Could you check a few things on this model? Use its own coordinates, in mm. Coordinates: 2 decimals unless noted, no trailing zeros. Write each loop counter-clockwise with the first axis right and the second up, starting at its lowest first coordinate (ties: lowest second). Pieces come first, ordered by that corner, then holes. Notation, with made-up numbers: M 15.25,7 L 39.25,7 A29 ccw 39.25,46 Z; hole C -31,84 d9. An arc over 180 degrees is marked long. Answer as CSV lines item,"result". Start each with the question number.
Item 1: We'd pull the mould along X, two halves only. Please class faces 1 (the cylindrical face through (137.02, -138.517, -0.744)), 2 (the cylindrical face through (137.528, -164.615, -0.744)), 3 (the flat face through (120, -106, 0)): +X half, -X half, draft (parallel to the pull), parting line (faces both ways), or undercut.
Item 2: Suppose I cut it at B-B, the plane y = -94. Write out the boundary of the cut face in (x, z).
Item 3: I'm going to push flat-ended pins straight in: P1, Ø0.5, axis at y = -149.5, z = -1, coming from the -X side; P2, Ø0.8, axis at y = -149, z = -1, coming from the +X side. Where does each tip first touch, or does it pass through?
Item 4: If I drill on line 1 along Y through (x, z) = (123, -1); line 2 along X through (y, z) = (-57, -1.05); line 3 along Y through (x, z) = (121.5, -1.35), over which ranges is the centre line in solid material (lowest first)? Write a range as [from, to].
Item 5: Suppose I cut it at A-A, the plane z = -0.4. State how many separate pieces and enclosed holes the cut face has, and give its area (3 significant figures).
```python
from build123d import *

# Parameters (mm, degrees)
SKETCH1_R           = 0.85
SKETCH1_R_2         = 2
SKETCH1_R_3         = 0.75
SKETCH1_R_4         = 1.1
BOSS_EXTRUDE1_DEPTH = 1.51


with BuildPart() as part:
    # Sketch1 → Boss-Extrude1 (new body)
    with BuildSketch(Plane.XY):
        with BuildLine():
            Line((136.512, -46.6938), (104.012, -46.6938))
            ThreePointArc((104.012, -46.6938), (101.512, -49.1938), (104.012, -51.6938))
            ThreePointArc((104.012, -51.6938), (105.779767, -52.426033), (106.512, -54.1938))
            Line((106.512, -54.1938), (106.512, -132.541))
            ThreePointArc((106.512, -132.541), (105.779767, -134.308767), (104.012, -135.041))
            ThreePointArc((104.012, -135.041), (101.512, -137.541), (104.012, -140.041))
            ThreePointArc((104.012, -140.041), (105.779767, -140.773233), (106.512, -142.541))
            Line((106.512, -142.541), (106.512, -159.1938))
            ThreePointArc((106.512, -159.1938), (105.779767, -160.961567), (104.012, -161.6938))
            ThreePointArc((104.012, -161.6938), (101.512, -164.1938), (104.012, -166.6938))
            Line((104.012, -166.6938), (136.512, -166.6938))
            ThreePointArc((136.512, -166.6938), (139.012, -164.1938), (136.512, -161.6938))
            ThreePointArc((136.512, -161.6938), (134.744233, -160.961567), (134.012, -159.1938))
            Line((134.012, -159.1938), (134.012, -142.541))
            ThreePointArc((134.012, -142.541), (134.744233, -140.773233), (136.512, -140.041))
            ThreePointArc((136.512, -140.041), (139.012, -137.541), (136.512, -135.041))
            ThreePointArc((136.512, -135.041), (134.744233, -134.308767), (134.012, -132.541))
            Line((134.012, -132.541), (134.012, -54.1938))
            ThreePointArc((134.012, -54.1938), (134.744233, -52.426033), (136.512, -51.6938))
            ThreePointArc((136.512, -51.6938), (139.012, -49.1938), (136.512, -46.6938))
        make_face()
        with Locations((125.603, -137.541)):
            Circle(SKETCH1_R, mode=Mode.SUBTRACT)
        with Locations((120.523, -137.541)):
            Circle(SKETCH1_R_2, mode=Mode.SUBTRACT)
        with Locations((115.443, -137.541)):
            Circle(SKETCH1_R, mode=Mode.SUBTRACT)
        with Locations((116.713, -140.081)):
            Circle(SKETCH1_R_3, mode=Mode.SUBTRACT)
        with Locations((123.063, -142.621)):
            Circle(SKETCH1_R_3, mode=Mode.SUBTRACT)
        with Locations((104.012, -137.541)):
            Circle(SKETCH1_R_4, mode=Mode.SUBTRACT)
        with Locations((104.012, -164.1938)):
            Circle(SKETCH1_R_4, mode=Mode.SUBTRACT)
        with Locations((136.512, -164.1938)):
            Circle(SKETCH1_R_4, mode=Mode.SUBTRACT)
        with Locations((136.512, -137.541)):
            Circle(SKETCH1_R_4, mode=Mode.SUBTRACT)
        with Locations((136.512, -49.1938)):
            Circle(SKETCH1_R_4, mode=Mode.SUBTRACT)
        with Locations((104.012, -49.1938)):
            Circle(SKETCH1_R_4, mode=Mode.SUBTRACT)
    extrude(amount=-BOSS_EXTRUDE1_DEPTH)


solid = part.part
```
Ans:
1,face 1,"undercut"
1,face 2,"undercut"
1,face 3,"draft"
2,outline,"M 106.51,-1.51 L 134.01,-1.51 L 134.01,0 L 106.51,0 Z"
3,P1,"stops at x = 106.51"
3,P2,"stops at x = 134.01"
4,line 1,"y = [-166.69, -143.37], [-141.87, -46.69]"
4,line 2,"x = [106.51, 134.01]"
4,line 3,"y = [-166.69, -139.29], [-135.8, -46.69]"
5,separate pieces,"1"
5,enclosed holes,"11"
5,area,"3,400 mm^2"
